```python
from build123d import *

# Parameters (mm, degrees)
BOSS_EXTRUDE1_DEPTH = 1.5875


with BuildPart() as part:
    # Sketch1 → Boss-Extrude1 (new body, symmetric)
    with BuildSketch(Plane(origin=(0, 0, 0), x_dir=(0, 0, -1), z_dir=(1, 0, 0))):
        Polygon((23.8125, 0), (23.8125, 3.175), (17.4625, 3.175), (12.7, 28.575), (4.7625, 28.575), (4.7625, 25.4), (-4.7625, 25.4), (-4.7625, 28.575), (-12.7, 28.575), (-17.4625, 0), (-17.4625, -2.54), (-7.8867, -2.54), (-7.8867, 0), (7.8867, 0), (7.8867, -2.54), (17.4625, -2.54), (17.4625, 0), align=None)
    extrude(amount=BOSS_EXTRUDE1_DEPTH, both=True)


solid = part.part
```
Source: CAD feature listing. Evaluate the final solid. Frame: model axes, mm. A direction names the side the tool comes from. Coordinates: 2 decimals unless noted, no trailing zeros. Write each loop counter-clockwise with the first axis right and the second up, starting at its lowest first coordinate (ties: lowest second). Pieces come first, ordered by that corner, then holes. Notation, with made-up numbers: (33.25, 56.25) -> (78.25, 56.25) arc R32 ccw to (78.25, 89.25) -> close; hole circle Ø5 at (5.25, -4). An arc over 180 degrees is marked (long way). Return JSON: item names as keys, results as strings. Group by question number.
1) Ray query, line 1 along Z through (x, y) = (-0.8, -1); line 2 along Y through (x, z) = (0.75, -4); line 3 along Z through (x, y) = (1.15, 27). Return the intervals inside material, ascending.
2) Mould query, pull axis Z, two halves, no side actions, for faces 5 (the face through (0.022, 15.697, -15.115)), 6 (the face through (0.022, 14.488, 15.048)), 7 (the face through (0, -2.54, 13)), 8 (the face through (0, 25.4, 0)). Classes: +Z half, -Z half, draft (parallel to the pull), parting line (faces both ways), or undercut.
3) Section query B-B, the plane z = 1. Return loops of the section in (x, y).
4) Section query A-A, the plane x = 0.8. Return loops of the section in (y, z) (1 decimal).
5) Section query C-C, the plane y = 10. Return loops of the section in (x, z), plus the area to 3 significant figures.
6) Set-up query: faces 1 (the face through (0, -1, -17.462)), 2 (the face through (0, 27, 4.762)), 3 (the face through (0, 3.175, -21)), 4 (the face through (0, -1, -7.887)). Return all of +Z, -Z, +X, -X, +Y, -Y with unobstructed straight access to the full face (end or side cutting, diameter ignored); none if empty.
7) Contact query for flat-ended pins moving along their axis: P1, Ø1, axis at x = -0.5, z = 2.5, coming from the +Y side; P2, Ø1.5, axis at x = 1, z = 0, coming from the -Y side; P3, Ø1, axis at x = 0, y = 26, coming from the +Z side. Output: stop coordinate, or through.
From the geometry:
{
 "1": {"line 1": "-17.46 to -7.89, 7.89 to 17.46", "line 2": "0 to 25.4", "line 3": "-13 to -4.76, 4.76 to 12.96"},
 "2": {"face 5": "-Z half", "face 6": "+Z half", "face 7": "draft", "face 8": "undercut"},
 "3": {"outline": "(-1.59, 0) -> (1.59, 0) -> (1.59, 25.4) -> (-1.59, 25.4) -> close"},
 "4": {"outline": "(-2.5, -17.5) -> (0, -17.5) -> (0, -23.8) -> (3.2, -23.8) -> (3.2, -17.5) -> (28.6, -12.7) -> (28.6, -4.8) -> (25.4, -4.8) -> (25.4, 4.8) -> (28.6, 4.8) -> (28.6, 12.7) -> (0, 17.5) -> (-2.5, 17.5) -> (-2.5, 7.9) -> (0, 7.9) -> (0, -7.9) -> (-2.5, -7.9) -> close"},
 "5": {"outline": "(-1.59, -16.18) -> (1.59, -16.18) -> (1.59, 15.8) -> (-1.59, 15.8) -> close", "area": "102 mm²"},
 "6": {"face 1": "-Z, +X, -X, -Y", "face 2": "+X, -X, +Y", "face 3": "-Z, +X, -X, +Y", "face 4": "+X, -X, -Y"},
 "7": {"P1": "y = 25.4", "P2": "y = 0", "P3": "z = 13.21"}
}
